Input: part model. Units: mm. Frame: model coordinates. A direction names the side the tool comes from. Round coordinates to 2 decimals unless told otherwise and drop trailing zeros. Loops run counter-clockwise (first coordinate to the right, second up) from the corner with the lowest first, then second, coordinate; pieces in that order, holes last. Notation, with made-up numbers: (-1, 21) -> (22, 21) arc R23 cw to (22, 39) -> close; hole circle Ø2 at (58.25, 18). An arc over 180 degrees is marked (long way). Answer as a JSON object with one key per item and string values. Group by question number.
Item 1: Material intervals for line 1 (Y direction, x = -8, z = 7); line 2 (X direction, y = -1, z = -2.5); line 3 (Z direction, x = 3.5, y = 13.5), sorted ascending. Write a range as [from, to].
Item 2: Section query A-A on z = -7.75. Return loops of the section in (x, y), and give its area (3 significant figures).
Item 3: Set-up query: faces 1 (the cylindrical face through (5.77, -11.09, 5.25)), 2 (the flat face through (0, 0, -13)), 3 (the cylindrical face through (-14.13, -8.01, -13.14)). Return all of +Z, -Z, +X, -X, +Y, -Y with unobstructed straight access to the full face (end or side cutting, diameter ignored); none if empty.
Item 4: Pin query (flat end, axial travel): pin 1 (1.5 mm diameter, centred on x = -11, z = -1.5, fed in from +Y); pin 2 (6 mm diameter, centred on y = 10, z = 4.5, fed in from -X); pin 3 (10 mm diameter, centred on y = -1, z = 10, fed in from -X). Return the tip coordinate at first contact, or that it passes through.
from build123d import *

# Parameters (mm, degrees)
SKETCH1_R           = 12.5
BOSS_EXTRUDE1_DEPTH = 13.29
SKETCH2_R           = 12.5
BOSS_EXTRUDE2_DEPTH = 13
BOSS_EXTRUDE3_START = 13.29
SKETCH2_2_R         = 12.5
BOSS_EXTRUDE3_DEPTH = 13.29
CHAMFER1_SIZE       = 3
FILLET1_R           = 1
FILLET2_R           = 0.5
FILLET3_R           = 0.5


with BuildPart() as part:
    # Sketch1 → Boss-Extrude1 (new body)
    with BuildSketch(Plane.XY):
        Polygon((18.918054635, 0), (9.459027317, 16.383515904), (-9.459027317, 16.383515904), (-18.918054635, 0), (-9.459027317, -16.383515904), (9.459027317, -16.383515904), align=None)
        Circle(SKETCH1_R, mode=Mode.SUBTRACT)
    extrude(amount=-BOSS_EXTRUDE1_DEPTH)

    # Sketch2 → Boss-Extrude2 (add)
    with BuildSketch(Plane.XY):
        Circle(SKETCH2_R)
    extrude(amount=-BOSS_EXTRUDE2_DEPTH)

    # Sketch2<2> → Boss-Extrude3 (add)
    with BuildSketch(Plane.XY.offset(BOSS_EXTRUDE3_START)):
        Circle(SKETCH2_2_R)
    extrude(amount=-BOSS_EXTRUDE3_DEPTH)

    # Chamfer1
    chamfer1_edges = [part.edges().sort_by_distance(p)[0] for p in [
        (-12.5, 0, 13.29),
    ]]
    chamfer(chamfer1_edges, length=CHAMFER1_SIZE)

    # Fillet1
    fillet1_edges = [part.edges().sort_by_distance(p)[0] for p in [
        (-9.5, 0, 13.29),
        (-12.5, 0, 10.29),
    ]]
    fillet(fillet1_edges, radius=FILLET1_R)

    # Fillet2
    # the kernel refuses this fillet: 0.5 mm, written as the material it takes off along each edge
    with BuildSketch(Plane(origin=(9.170352183, -15.883515904, -0.5), x_dir=(0.866025403784439, -0.4999999999999994, 0), z_dir=(0, 0, 1))) as fillet2_piece_1_section:
        Polygon((0, 0), (FILLET2_R * 1.02, 0), (FILLET2_R * 1.02, -FILLET2_R * 0.588897274573), (FILLET2_R * 0.51, -FILLET2_R * 0.88334591186), align=None)
    fillet2_piece_1 = extrude(amount=FILLET2_R * 1.02, mode=Mode.PRIVATE)
    fillet2_piece_1 = fillet2_piece_1 - Plane(origin=(9.170352183, -15.883515904, -0.5), x_dir=(-0.5000000000000004, 0.8660254037844384, 0), z_dir=(0, 0, 1)) * Sphere(FILLET2_R, mode=Mode.PRIVATE)
    add(fillet2_piece_1, mode=Mode.SUBTRACT)
    with BuildSketch(Plane(origin=(9.170352183, -15.883515904, -12.79), x_dir=(0.866025403784439, -0.4999999999999994, 0), z_dir=(0, 0, -1))) as fillet2_piece_2_section:
        Polygon((0, 0), (FILLET2_R * 1.02, 0), (FILLET2_R * 1.02, FILLET2_R * 0.588897274573), (FILLET2_R * 0.51, FILLET2_R * 0.88334591186), align=None)
    fillet2_piece_2 = extrude(amount=FILLET2_R * 1.02, mode=Mode.PRIVATE)
    fillet2_piece_2 = fillet2_piece_2 - Plane(origin=(9.170352183, -15.883515904, -12.79), x_dir=(-0.5000000000000004, 0.8660254037844384, 0), z_dir=(0, 0, -1)) * Sphere(FILLET2_R, mode=Mode.PRIVATE)
    add(fillet2_piece_2, mode=Mode.SUBTRACT)
    with BuildSketch(Plane(origin=(-9.170352183, -15.883515904, -0.5), x_dir=(0, -1, 0), z_dir=(0, 0, 1))) as fillet2_piece_3_section:
        Polygon((0, 0), (FILLET2_R * 1.02, 0), (FILLET2_R * 1.02, -FILLET2_R * 0.588897274573), (FILLET2_R * 0.51, -FILLET2_R * 0.88334591186), align=None)
    fillet2_piece_3 = extrude(amount=FILLET2_R * 1.02, mode=Mode.PRIVATE)
    fillet2_piece_3 = fillet2_piece_3 - Plane(origin=(-9.170352183, -15.883515904, -0.5), x_dir=(0.49999999999999983, 0.8660254037844387, 0), z_dir=(0, 0, 1)) * Sphere(FILLET2_R, mode=Mode.PRIVATE)
    add(fillet2_piece_3, mode=Mode.SUBTRACT)
    with BuildSketch(Plane(origin=(-9.170352183, -15.883515904, -12.79), x_dir=(0, -1, 0), z_dir=(0, 0, -1))) as fillet2_piece_4_section:
        Polygon((0, 0), (FILLET2_R * 1.02, 0), (FILLET2_R * 1.02, FILLET2_R * 0.588897274573), (FILLET2_R * 0.51, FILLET2_R * 0.88334591186), align=None)
    fillet2_piece_4 = extrude(amount=FILLET2_R * 1.02, mode=Mode.PRIVATE)
    fillet2_piece_4 = fillet2_piece_4 - Plane(origin=(-9.170352183, -15.883515904, -12.79), x_dir=(0.49999999999999983, 0.8660254037844387, 0), z_dir=(0, 0, -1)) * Sphere(FILLET2_R, mode=Mode.PRIVATE)
    add(fillet2_piece_4, mode=Mode.SUBTRACT)
    with BuildSketch(Plane(origin=(-18.340704365, 0, -0.5), x_dir=(-0.8660254037844388, 0.49999999999999967, 0), z_dir=(0, 0, 1))) as fillet2_piece_5_section:
        Polygon((0, 0), (FILLET2_R * 1.02, 0), (FILLET2_R * 1.02, FILLET2_R * 0.588897274573), (FILLET2_R * 0.51, FILLET2_R * 0.88334591186), align=None)
    fillet2_piece_5 = extrude(amount=FILLET2_R * 1.02, mode=Mode.PRIVATE)
    fillet2_piece_5 = fillet2_piece_5 - Plane(origin=(-18.340704365, 0, -0.5), x_dir=(1, 0, 0), z_dir=(0, 0, 1)) * Sphere(FILLET2_R, mode=Mode.PRIVATE)
    add(fillet2_piece_5, mode=Mode.SUBTRACT)
    with BuildSketch(Plane(origin=(-18.340704365, 0, -12.79), x_dir=(-0.8660254037844388, 0.49999999999999967, 0), z_dir=(0, 0, -1))) as fillet2_piece_6_section:
        Polygon((0, 0), (FILLET2_R * 1.02, 0), (FILLET2_R * 1.02, -FILLET2_R * 0.588897274573), (FILLET2_R * 0.51, -FILLET2_R * 0.88334591186), align=None)
    fillet2_piece_6 = extrude(amount=FILLET2_R * 1.02, mode=Mode.PRIVATE)
    fillet2_piece_6 = fillet2_piece_6 - Plane(origin=(-18.340704365, 0, -12.79), x_dir=(1, 0, 0), z_dir=(0, 0, -1)) * Sphere(FILLET2_R, mode=Mode.PRIVATE)
    add(fillet2_piece_6, mode=Mode.SUBTRACT)
    with BuildSketch(Plane(origin=(-9.170352183, 15.883515904, -0.5), x_dir=(0, 1, 0), z_dir=(0, 0, 1))) as fillet2_piece_7_section:
        Polygon((0, 0), (FILLET2_R * 1.02, 0), (FILLET2_R * 1.02, FILLET2_R * 0.588897274573), (FILLET2_R * 0.51, FILLET2_R * 0.88334591186), align=None)
    fillet2_piece_7 = extrude(amount=FILLET2_R * 1.02, mode=Mode.PRIVATE)
    fillet2_piece_7 = fillet2_piece_7 - Plane(origin=(-9.170352183, 15.883515904, -0.5), x_dir=(0.5000000000000002, -0.8660254037844386, 0), z_dir=(0, 0, 1)) * Sphere(FILLET2_R, mode=Mode.PRIVATE)
    add(fillet2_piece_7, mode=Mode.SUBTRACT)
    with BuildSketch(Plane(origin=(-9.170352183, 15.883515904, -12.79), x_dir=(0, 1, 0), z_dir=(0, 0, -1))) as fillet2_piece_8_section:
        Polygon((0, 0), (FILLET2_R * 1.02, 0), (FILLET2_R * 1.02, -FILLET2_R * 0.588897274573), (FILLET2_R * 0.51, -FILLET2_R * 0.88334591186), align=None)
    fillet2_piece_8 = extrude(amount=FILLET2_R * 1.02, mode=Mode.PRIVATE)
    fillet2_piece_8 = fillet2_piece_8 - Plane(origin=(-9.170352183, 15.883515904, -12.79), x_dir=(0.5000000000000002, -0.8660254037844386, 0), z_dir=(0, 0, -1)) * Sphere(FILLET2_R, mode=Mode.PRIVATE)
    add(fillet2_piece_8, mode=Mode.SUBTRACT)
    with BuildSketch(Plane(origin=(9.170352183, 15.883515904, -0.5), x_dir=(0.8660254037844384, 0.5000000000000006, 0), z_dir=(0, 0, 1))) as fillet2_piece_9_section:
        Polygon((0, 0), (FILLET2_R * 1.02, 0), (FILLET2_R * 1.02, FILLET2_R * 0.588897274573), (FILLET2_R * 0.51, FILLET2_R * 0.88334591186), align=None)
    fillet2_piece_9 = extrude(amount=FILLET2_R * 1.02, mode=Mode.PRIVATE)
    fillet2_piece_9 = fillet2_piece_9 - Plane(origin=(9.170352183, 15.883515904, -0.5), x_dir=(-0.4999999999999997, -0.8660254037844387, 0), z_dir=(0, 0, 1)) * Sphere(FILLET2_R, mode=Mode.PRIVATE)
    add(fillet2_piece_9, mode=Mode.SUBTRACT)
    with BuildSketch(Plane(origin=(9.170352183, 15.883515904, -12.79), x_dir=(0.8660254037844384, 0.5000000000000006, 0), z_dir=(0, 0, -1))) as fillet2_piece_10_section:
        Polygon((0, 0), (FILLET2_R * 1.02, 0), (FILLET2_R * 1.02, -FILLET2_R * 0.588897274573), (FILLET2_R * 0.51, -FILLET2_R * 0.88334591186), align=None)
    fillet2_piece_10 = extrude(amount=FILLET2_R * 1.02, mode=Mode.PRIVATE)
    fillet2_piece_10 = fillet2_piece_10 - Plane(origin=(9.170352183, 15.883515904, -12.79), x_dir=(-0.4999999999999997, -0.8660254037844387, 0), z_dir=(0, 0, -1)) * Sphere(FILLET2_R, mode=Mode.PRIVATE)
    add(fillet2_piece_10, mode=Mode.SUBTRACT)
    with BuildSketch(Plane(origin=(18.340704365, 0, -0.5), x_dir=(0.8660254037844384, 0.5000000000000006, 0), z_dir=(0, 0, 1))) as fillet2_piece_11_section:
        Polygon((0, 0), (FILLET2_R * 1.02, 0), (FILLET2_R * 1.02, -FILLET2_R * 0.588897274573), (FILLET2_R * 0.51, -FILLET2_R * 0.88334591186), align=None)
    fillet2_piece_11 = extrude(amount=FILLET2_R * 1.02, mode=Mode.PRIVATE)
    fillet2_piece_11 = fillet2_piece_11 - Plane(origin=(18.340704365, 0, -0.5), x_dir=(-1, 0, 0), z_dir=(0, 0, 1)) * Sphere(FILLET2_R, mode=Mode.PRIVATE)
    add(fillet2_piece_11, mode=Mode.SUBTRACT)
    with BuildSketch(Plane(origin=(18.340704365, 0, -12.79), x_dir=(0.8660254037844384, 0.5000000000000006, 0), z_dir=(0, 0, -1))) as fillet2_piece_12_section:
        Polygon((0, 0), (FILLET2_R * 1.02, 0), (FILLET2_R * 1.02, FILLET2_R * 0.588897274573), (FILLET2_R * 0.51, FILLET2_R * 0.88334591186), align=None)
    fillet2_piece_12 = extrude(amount=FILLET2_R * 1.02, mode=Mode.PRIVATE)
    fillet2_piece_12 = fillet2_piece_12 - Plane(origin=(18.340704365, 0, -12.79), x_dir=(-1, 0, 0), z_dir=(0, 0, -1)) * Sphere(FILLET2_R, mode=Mode.PRIVATE)
    add(fillet2_piece_12, mode=Mode.SUBTRACT)
    with BuildSketch(Plane(origin=(9.459027317, -16.383515904, -0.5), x_dir=(0.499999999999998, 0.8660254037844398, 0), z_dir=(0, 0, -1)), Plane(origin=(-9.459027317, -16.383515904, -0.5), x_dir=(1, 0, 0), z_dir=(0, 0, -1)), Plane(origin=(18.918054635, 0, -0.5), x_dir=(-0.500000000000001, 0.8660254037844382, 0), z_dir=(0, 0, -1))) as fillet2_piece_13:
        with BuildLine():
            CenterArc((FILLET2_R * 0.57735026919, -FILLET2_R), FILLET2_R, 90, 60)
            Line((-FILLET2_R * 0.288675134595, -FILLET2_R * 0.5), (-FILLET2_R * 0.305995642671, -FILLET2_R * 0.49))
            Line((-FILLET2_R * 0.305995642671, -FILLET2_R * 0.49), (-FILLET2_R * 0.0115470053838, FILLET2_R * 0.02))
            Line((-FILLET2_R * 0.0115470053838, FILLET2_R * 0.02), (FILLET2_R * 0.57735026919, FILLET2_R * 0.02))
            Line((FILLET2_R * 0.57735026919, FILLET2_R * 0.02), (FILLET2_R * 0.57735026919, 0))
        make_face()
    extrude(amount=12.29, mode=Mode.SUBTRACT)
    with BuildSketch(Plane(origin=(-18.918054635, 0, -0.5), x_dir=(0.49999999999999345, 0.8660254037844424, 0), z_dir=(0, 0, -1)), Plane(origin=(-9.459027317, 16.383515904, -0.5), x_dir=(1, 0, 0), z_dir=(0, 0, -1)), Plane(origin=(9.459027317, 16.383515904, -0.5), x_dir=(0.499999999999998, -0.8660254037844398, 0), z_dir=(0, 0, -1))) as fillet2_piece_14:
        with BuildLine():
            CenterArc((FILLET2_R * 0.57735026919, FILLET2_R), FILLET2_R, 210, 60)
            Line((-FILLET2_R * 0.288675134595, FILLET2_R * 0.5), (-FILLET2_R * 0.30599564267, FILLET2_R * 0.49))
            Line((-FILLET2_R * 0.30599564267, FILLET2_R * 0.49), (-FILLET2_R * 0.0115470053838, -FILLET2_R * 0.02))
            Line((-FILLET2_R * 0.0115470053838, -FILLET2_R * 0.02), (FILLET2_R * 0.57735026919, -FILLET2_R * 0.02))
            Line((FILLET2_R * 0.57735026919, -FILLET2_R * 0.02), (FILLET2_R * 0.57735026919, 0))
        make_face()
    extrude(amount=12.29, mode=Mode.SUBTRACT)
    with BuildSketch(Plane(origin=(9.170352183, 16.383515904, -13.29), x_dir=(0, 0, 1), z_dir=(-1, 0, 0)), Plane(origin=(-9.603364885, 16.133515904, -13.29), x_dir=(0, 0, 1), z_dir=(-0.4999999999999997, -0.8660254037844389, 0)), Plane(origin=(-18.773717067, -0.25, -13.29), x_dir=(0, 0, 1), z_dir=(0.5000000000000002, -0.8660254037844386, 0)), Plane(origin=(-9.170352183, -16.383515904, -13.29), x_dir=(0, 0, 1), z_dir=(1, 0, 0)), Plane(origin=(9.603364885, -16.133515904, -13.29), x_dir=(0, 0, 1), z_dir=(0.4999999999999994, 0.866025403784439, 0)), Plane(origin=(-9.170352183, -16.383515904, 0), x_dir=(0, 1, 0), z_dir=(1, 0, 0)), Plane(origin=(-18.773717067, -0.25, 0), x_dir=(0.8660254037844386, 0.5000000000000002, 0), z_dir=(0.5000000000000002, -0.8660254037844386, 0)), Plane(origin=(-9.603364885, 16.133515904, 0), x_dir=(0.8660254037844388, -0.49999999999999967, 0), z_dir=(-0.4999999999999997, -0.8660254037844389, 0)), Plane(origin=(9.170352183, 16.383515904, 0), x_dir=(0, -1, 0), z_dir=(-1, 0, 0)), Plane(origin=(18.773717067, 0.25, 0), x_dir=(-0.8660254037844384, -0.5000000000000006, 0), z_dir=(-0.5000000000000006, 0.8660254037844384, 0)), Plane(origin=(9.603364885, -16.133515904, 0), x_dir=(-0.866025403784439, 0.49999999999999933, 0), z_dir=(0.4999999999999994, 0.866025403784439, 0)), Plane(origin=(18.773717067, 0.25, -13.29), x_dir=(0, 0, 1), z_dir=(-0.5000000000000006, 0.8660254037844384, 0))) as fillet2_piece_15:
        with BuildLine():
            CenterArc((FILLET2_R, -FILLET2_R), FILLET2_R, 90, 90)
            Line((0, -FILLET2_R), (-FILLET2_R * 0.02, -FILLET2_R))
            Line((-FILLET2_R * 0.02, -FILLET2_R), (-FILLET2_R * 0.02, FILLET2_R * 0.02))
            Line((-FILLET2_R * 0.02, FILLET2_R * 0.02), (FILLET2_R, FILLET2_R * 0.02))
            Line((FILLET2_R, FILLET2_R * 0.02), (FILLET2_R, 0))
        make_face()
    extrude(amount=18.340704365, mode=Mode.SUBTRACT)
    with BuildSketch(Plane(origin=(0, 0, -13.29), x_dir=(1, 0, 0), z_dir=(0, -1, 0))) as fillet2_piece_16:
        with BuildLine():
            CenterArc((12.953762052, 0.5), FILLET2_R, 204.83458749, 65.16541251)
            Line((12.5, 0.29), (12.490924759, 0.2858))
            ThreePointArc((12.490924759, 0.2858), (12.49, 0.145), (12.49, 0))
            Line((12.49, 0), (12.5, -0.01))
            Line((12.5, -0.01), (12.953762052, -0.01))
            Line((12.953762052, -0.01), (12.953762052, 0))
        make_face()
    revolve(axis=Axis((0, 0, -13.29), (0, 0, 1)), mode=Mode.SUBTRACT)

    # Fillet3
    fillet3_edges = [part.edges().sort_by_distance(p)[0] for p in [
        (-12.5, 0, 0),
    ]]
    fillet(fillet3_edges, radius=FILLET3_R)


solid = part.part
Solved:
{
 "1": {"line 1": "[-9.6, 9.6]", "line 2": "[-18.34, 18.34]", "line 3": "[-13.29, 0]"},
 "2": {"outline": "(-18.77, -0.25) -> (-9.6, -16.13) arc R0.5 ccw to (-9.17, -16.38) -> (9.17, -16.38) arc R0.5 ccw to (9.6, -16.13) -> (18.77, -0.25) arc R0.5 ccw to (18.77, 0.25) -> (9.6, 16.13) arc R0.5 ccw to (9.17, 16.38) -> (-9.17, 16.38) arc R0.5 ccw to (-9.6, 16.13) -> (-18.77, 0.25) arc R0.5 ccw to start", "area": "930 mm²"},
 "3": {"face 1": "+Z", "face 2": "-Z", "face 3": "-Z, -X, -Y"},
 "4": {"pin 1": "y = 15.01", "pin 2": "x = -10.36", "pin 3": "x = -12.5"}
}
